Geometry: final body of the model. Coordinates: model frame, mm. A direction names the side the tool comes from. Give positions to 0.01 mm unless a question says otherwise; leave off trailing zeros. Write each loop counter-clockwise with the first axis right and the second up, starting at its lowest first coordinate (ties: lowest second). Pieces come first, ordered by that corner, then holes. Notation, with made-up numbers: (-19.5, 32) -> (-15.5, 32) arc R17 ccw to (-15.5, 64) -> close; hole circle Ø9 at (50, -19.5). An arc over 180 degrees is marked (long way). Answer as a JSON object with one key per item and string values. Group by question number.
(1) Section query C-C on z = -7.25. Output: boundary loops of the cut face in (x, y), plus the area to 3 significant figures.
(2) Section query A-A on y = 4. Output: boundary loops of the cut face in (x, z).
(3) Section query B-B on y = 6.5. Output: boundary loops of the cut face in (x, z).
(4) Contact query for flat-ended pins moving along their axis: pin 1 Ø2 at (x, z) = (-19.5, -6) entering from -Y; pin 2 Ø1.5 at (x, z) = (27, -5) entering from -Y; pin 3 Ø10 at (x, y) = (7, 7.5) entering from -Z. Output: stop coordinate, or through.
(5) Section query D-D on x = -7. Output: boundary loops of the cut face in (y, z), plus the area to 3 significant figures.
(6) Draft query along X for faces 4 (the face through (-27, 5, -5)), 5 (the face through (-32.5, 6, -5)), 6 (the face through (0, 17, -10)). Return one class per face: +X half, -X half, draft (parallel to the pull), parting line (faces both ways), or undercut.
(7) Set-up query: faces 1 (the face through (-22.5, 8, -5)), 2 (the face through (-26, 2, -5)), 3 (the face through (26, 0, -6)). Return all of +Z, -Z, +X, -X, +Y, -Y with unobstructed straight access to the full face (end or side cutting, diameter ignored); none if empty.
(8) Material intervals for probe 1 along X at (y, z) = (2.05, -5); probe 2 along X at (y, z) = (4.75, -7.5); probe 3 along Y at (x, z) = (-13, -6.75), sorted ascending.
from build123d import *

# Parameters (mm, degrees)
CROQUIS1_W                = 10
CROQUIS1_H                = 10
SALIENTE_EXTRUIR1_DEPTH   = 15.5
SALIENTE_EXTRUIR1_2_DEPTH = 15.5
CROQUIS5_W                = 65
CROQUIS5_H                = 10
SALIENTE_EXTRUIR4_DEPTH   = 2
CROQUIS6_R                = 1.5
CORTAR_EXTRUIR2_DEPTH     = 5
REDONDEO1_R               = 5


with BuildPart() as part:
    # Croquis1 → Saliente-Extruir1 (new body)
    with BuildSketch(Plane(origin=(0, 0, 0), x_dir=(1, 0, 0), z_dir=(0, 1, 0))):
        with Locations((-27.5, 5)):
            Rectangle(CROQUIS1_W, CROQUIS1_H)
    extrude(amount=SALIENTE_EXTRUIR1_DEPTH)



with BuildPart() as body_2:
    # Croquis1 → Saliente-Extruir1 2 (new body)
    with BuildSketch(Plane(origin=(0, 0, 0), x_dir=(1, 0, 0), z_dir=(0, 1, 0))):
        with Locations((27.5, 5)):
            Rectangle(CROQUIS1_W, CROQUIS1_H)
    extrude(amount=SALIENTE_EXTRUIR1_2_DEPTH)


with BuildPart() as part_1:
    add(part.part)

    add(body_2.part)  # Saliente-Extruir4 merges body 2
    # Croquis5 → Saliente-Extruir4 (add)
    with BuildSketch(Plane(origin=(0, 15.5, 0), x_dir=(1, 0, 0), z_dir=(0, 1, 0))):
        with Locations((0, 5)):
            Rectangle(CROQUIS5_W, CROQUIS5_H)
    extrude(amount=SALIENTE_EXTRUIR4_DEPTH)

    # Croquis6 → Cortar-Extruir2 (cut)
    with BuildSketch(Plane.XZ):
        with Locations(Location((-27.5, -5, 0), (0, 0, 270))):
            Circle(CROQUIS6_R)
        with Locations(Location((27.5, -5, 0), (0, 0, 270))):
            Circle(CROQUIS6_R)
    extrude(amount=-CORTAR_EXTRUIR2_DEPTH, mode=Mode.SUBTRACT)

    # Redondeo1
    redondeo1_edges = [part_1.edges().sort_by_distance(p)[0] for p in [
        (-32.5, 17.5, -5),
        (32.5, 17.5, -5),
    ]]
    fillet(redondeo1_edges, radius=REDONDEO1_R)


solid = part_1.part
Answer list:
{
 "1": {"outline": "(-32.5, 0) -> (-22.5, 0) -> (-22.5, 15.5) -> (22.5, 15.5) -> (22.5, 0) -> (32.5, 0) -> (32.5, 12.5) arc R5 ccw to (27.5, 17.5) -> (-27.5, 17.5) arc R5 ccw to (-32.5, 12.5) -> close", "area": "429 mm2"},
 "2": {"outline": "(-32.5, -10) -> (-22.5, -10) -> (-22.5, 0) -> (-32.5, 0) -> close; (22.5, -10) -> (32.5, -10) -> (32.5, 0) -> (22.5, 0) -> close; hole circle Ø3 at (-27.5, -5); hole circle Ø3 at (27.5, -5)"},
 "3": {"outline": "(-32.5, -10) -> (-22.5, -10) -> (-22.5, 0) -> (-32.5, 0) -> close; (22.5, -10) -> (32.5, -10) -> (32.5, 0) -> (22.5, 0) -> close"},
 "4": {"pin 1": "y = 15.5", "pin 2": "y = 5", "pin 3": "through"},
 "5": {"outline": "(15.5, -10) -> (17.5, -10) -> (17.5, 0) -> (15.5, 0) -> close", "area": "20.0 mm2"},
 "6": {"face 4": "undercut", "face 5": "-X half", "face 6": "draft"},
 "7": {"face 1": "+Z, -Z, -Y", "face 2": "-Y", "face 3": "+Z, -Z, +X, -X, -Y"},
 "8": {"probe 1": "-32.5 to -29, -26 to -22.5, 22.5 to 26, 29 to 32.5", "probe 2": "-32.5 to -22.5, 22.5 to 32.5", "probe 3": "15.5 to 17.5"}
}
